The listing builds one solid part. Answer for the finished solid, in the listing's coordinates (mm). A direction names the side the tool comes from. Round coordinates to 2 decimals unless told otherwise and drop trailing zeros. Loops run counter-clockwise (first coordinate to the right, second up) from the corner with the lowest first, then second, coordinate; pieces in that order, holes last. Notation, with made-up numbers: (48.25, -39.75) -> (57.25, -39.75) arc R29 ccw to (57.25, -9.75) -> close; hole circle Ø1 at (11.5, 39). An arc over 180 degrees is marked (long way). Use a Markdown table: item, result. Add a question column.
Q1. Which of the six approach directions +Z, -Z, +X, -X, +Y, -Y give full straight-line access (tool end or side, diameter ignored) to faces 1 (the flat face through (20, 5, -50)), 2 (the flat face through (115, -25, -2)), 3 (the flat face through (-120, -50, 2))?
Q2. For a pull along Z with two mould halves and no side action, classify faces 4 (the flat face through (-115, -25, -2)), 5 (the flat face through (-1, 2, 150)), 6 (the flat face through (30, 5, -70)), 7 (the flat face through (-1, 2, -150)) as released by +Z, released by -Z, zero draft, split by the parting line, or undercut.
Q3. Section C-C on z = -36.5 is taken. Give the vertices of the cut face in (x, y), then the cut area to 3 significant figures.
Q4. Consider line 1 (X direction, y = -8, z = -44); line 2 (Y direction, x = -104.5, z = 54). Determine where each line is inside the solid, lowest interval first.
Q5. Section D-D on x = -97 is taken. Give the vertices of the cut face in (y, z), then the cut area to 3 significant figures.
Q6. Section B-B on z = -76 is taken. Give the vertices of the cut face in (x, y).
Q7. Given pin 1 Ø5 at (x, z) = (-76.5, -103.5) entering from -Y; pin 2 Ø6 at (x, y) = (72, -5.5) entering from +Z; pin 3 Ø10 at (x, y) = (-43, -2.5) entering from -Z, each flat-ended and moving along its own axis, determine where each tip first touches the part or whether it passes through.
Q8. Section A-A on y = -37 is taken. Give the vertices of the cut face in (x, z), then the cut area to 3 significant figures.
from build123d import *

# Parameters (mm, degrees)
SKETCH1_W           = 250
SKETCH1_H           = 300
SKETCH1_W_2         = 20
SKETCH1_H_2         = 40
BOSS_EXTRUDE1_DEPTH = 10
SKETCH2_W           = 10
SKETCH2_H           = 300
BOSS_EXTRUDE2_DEPTH = 50


with BuildPart() as part:
    # Sketch1 → Boss-Extrude1 (new body)
    with BuildSketch(Plane(origin=(0, 0, 0), x_dir=(1, 0, 0), z_dir=(0, 1, 0))):
        Rectangle(SKETCH1_W, SKETCH1_H)
        with Locations((30, 50)):
            Rectangle(SKETCH1_W_2, SKETCH1_H_2, mode=Mode.SUBTRACT)
    extrude(amount=BOSS_EXTRUDE1_DEPTH)

    # Sketch2 → Boss-Extrude2 (add)
    with BuildSketch(Plane.XZ):
        with Locations((120, 0)):
            Rectangle(SKETCH2_W, SKETCH2_H)
        with Locations((-120, 0)):
            Rectangle(SKETCH2_W, SKETCH2_H)
    extrude(amount=BOSS_EXTRUDE2_DEPTH)


solid = part.part
Checked values:
| question | item | result |
|---|---|---|
| 1 | face 1 | +Y, -Y |
| 1 | face 2 | +Z, -Z, -Y |
| 1 | face 3 | +Z, -Z, +X, -X, -Y |
| 2 | face 4 | zero draft |
| 2 | face 5 | released by +Z |
| 2 | face 6 | undercut |
| 2 | face 7 | released by -Z |
| 3 | outline | (-125, -50) -> (-115, -50) -> (-115, 0) -> (20, 0) -> (20, 10) -> (-125, 10) -> close; (40, 0) -> (115, 0) -> (115, -50) -> (125, -50) -> (125, 10) -> (40, 10) -> close |
| 3 | area | 3,300 mm2 |
| 4 | line 1 | x = -125 to -115, 115 to 125 |
| 4 | line 2 | y = 0 to 10 |
| 5 | outline | (0, -150) -> (10, -150) -> (10, 150) -> (0, 150) -> close |
| 5 | area | 3,000 mm2 |
| 6 | outline | (-125, -50) -> (-115, -50) -> (-115, 0) -> (115, 0) -> (115, -50) -> (125, -50) -> (125, 10) -> (-125, 10) -> close |
| 7 | pin 1 | stops at y = 0 |
| 7 | pin 2 | passes through |
| 7 | pin 3 | stops at z = -150 |
| 8 | outline | (-125, -150) -> (-115, -150) -> (-115, 150) -> (-125, 150) -> close; (115, -150) -> (125, -150) -> (125, 150) -> (115, 150) -> close |
| 8 | area | 6,000 mm2 |
